Could you check a few things on this drawing? It's one solid part, dimensions in mm from its lowest x, y, z. A direction names the side the tool comes from. Coordinates: 2 decimals unless noted, no trailing zeros. Order: outer loops, then holes, each group sorted by start corner. A loop starts at its lowest first (then second) coordinate and runs counter-clockwise, first axis right, second up. Notation, with made-up numbers: M 8.25,76 L 30.25,76 A21 ccw 30.25,113 Z; hole C 29.25,-35 d2. An arc over 180 degrees is marked long. One line per question, with ' | ' between items. Start each with the question number.
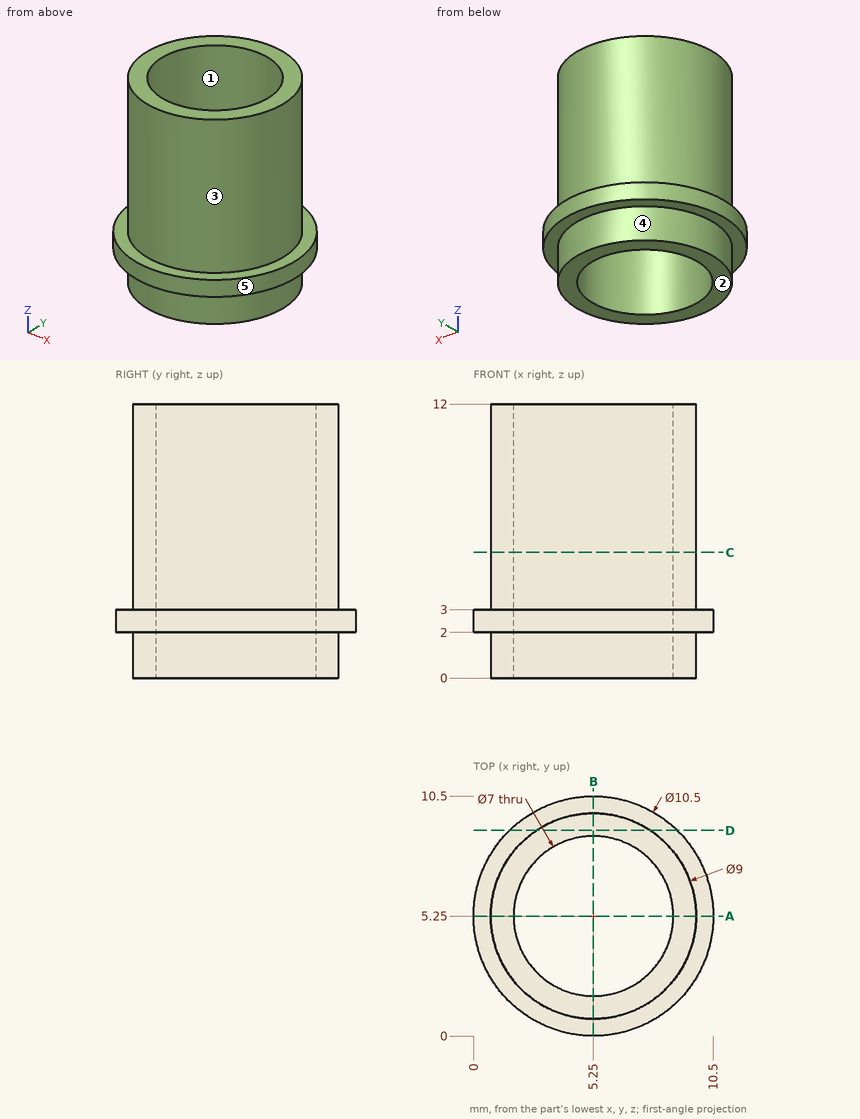
1. I need wall thicknesses on line 1 (Y direction, x = 5.25, z = 2.5); line 2 (Y direction, x = 5.25, z = 7.25); line 3 (X direction, y = 6.5, z = 10.5). Which ranges of each line are inside material? Lowest first, please.
2. Imagine slicing it at C-C (z = 5.5). List the corners of the cut face in (x, y) for me, then the cut area to 3 significant figures.
3. Imagine slicing it at A-A (y = 5.25). List the corners of the cut face in (x, z) for me, then the cut area to 3 significant figures.
4. Imagine slicing it at D-D (y = 9). List the corners of the cut face in (x, z) for me.
5. Will these pins go through, and if not, where does the flat tip stop? pin 1 (3 mm diameter, centred on x = 3, y = 8, fed in from -Z); pin 2 (1 mm diameter, centred on x = 4, y = 7, fed in from -Z); pin 3 (1.5 mm diameter, centred on x = 2.5, z = 3.5, fed in from +Y); pin 4 (1 mm diameter, centred on y = 8, z = 10.5, fed in from +X).
6. We'd pull the mould along Y, two halves only. Please class the marked faces 1, 2 and 3: released by +Y, released by -Y, zero draft, split by the parting line, or undercut.
7. Which directions (+Z, -Z, +X, -X, +Y, -Y) give clear straight access to the entire face, cutting with the end or side of a thin tool? Please do the marked faces 4 and 5.
Entries:
1) line 1: 0 to 1.75, 8.75 to 10.5 | line 2: 0.75 to 1.75, 8.75 to 9.75 | line 3: 0.93 to 1.98, 8.52 to 9.57
2) outline: C 5.25,5.25 d9; hole C 5.25,5.25 d7 | area: 25.1 mm²
3) outline: M 0,2 L 0.75,2 L 0.75,0 L 1.75,0 L 1.75,12 L 0.75,12 L 0.75,3 L 0,3 Z; M 8.75,0 L 9.75,0 L 9.75,2 L 10.5,2 L 10.5,3 L 9.75,3 L 9.75,12 L 8.75,12 Z | area: 25.5 mm²
4) outline: M 1.58,2 L 2.76,2 L 2.76,0 L 7.74,0 L 7.74,2 L 8.92,2 L 8.92,3 L 7.74,3 L 7.74,12 L 2.76,12 L 2.76,3 L 1.58,3 Z
5) pin 1: z = 0 | pin 2: through | pin 3: y = 10.02 | pin 4: x = 9.15
6) face 1: undercut | face 2: zero draft | face 3: split by the parting line
7) face 4: -Z | face 5: +Z, -Z
